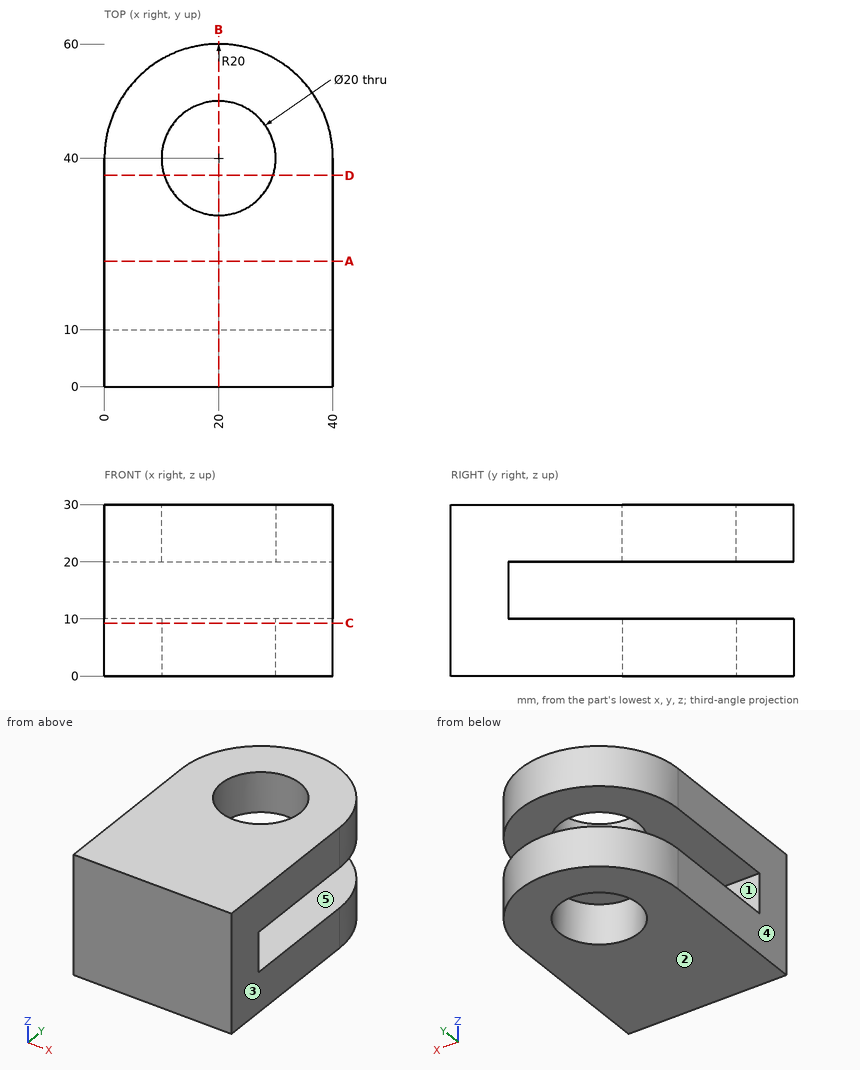
Answer from the drawing. Dimensions are ordinates in mm from the lowest x, y and z of the part. A direction names the side the tool comes from. Round coordinates to 2 decimals unless told otherwise and drop trailing zeros. Loops run counter-clockwise (first coordinate to the right, second up) from the corner with the lowest first, then second, coordinate; pieces in that order, holes last.
Q1. Section A-A on y = 22 is taken. Write down the section's boundary in (x, z).
Q2. Determine the mould class of the marked faces 1, 2 and 3 for opening direction Z: released by +Z, released by -Z, zero draft, split by the parting line, or undercut.
Q3. Consider probe 1 along Z at (x, y) = (21.5, 12); probe 2 along Y at (x, z) = (20, 4.75); probe 3 along X at (y, z) = (35.5, 21.25). Determine where each line is inside the solid, lowest interval first.
Q4. Section B-B on x = 20 is taken. Write down the section's boundary in (y, z).
Q5. Which of the six approach directions +Z, -Z, +X, -X, +Y, -Y give full straight-line access (tool end or side, diameter ignored) to the marked faces 4 and 5?
Q6. Section D-D on y = 37 is taken. Write down the section's boundary in (x, z), and give its area (3 significant figures).
Q7. Section C-C on z = 9.25 is taken. Write down the section's boundary in (x, y), and give its area (3 significant figures).
Q8. Each of these flat-tipped pins is pushed along its axis until it touches: pin 1 (12 mm diameter, centred on x = 20, y = 40, fed in from +Z); pin 2 (8 mm diameter, centred on x = 23.5, z = 15.5, fed in from +Y); pin 3 (10 mm diameter, centred on x = 16.5, z = 26, fed in from +Y). Where does it stop, or does it pass through?
Output:
1. outline: (0, 0) - (40, 0) - (40, 10) - (0, 10) - close; (0, 20) - (40, 20) - (40, 30) - (0, 30) - close
2. face 1: undercut
2. face 2: released by -Z
2. face 3: zero draft
3. probe 1: z = 0 to 10, 20 to 30
3. probe 2: y = 0 to 30, 50 to 60
3. probe 3: x = 0 to 11.07, 28.93 to 40
4. outline: (0, 0) - (30, 0) - (30, 10) - (10, 10) - (10, 20) - (30, 20) - (30, 30) - (0, 30) - close; (50, 0) - (60, 0) - (60, 10) - (50, 10) - close; (50, 20) - (60, 20) - (60, 30) - (50, 30) - close
5. face 4: +Z, -Z, -X, +Y, -Y
5. face 5: +X, -X, +Y
6. outline: (0, 0) - (10.46, 0) - (10.46, 10) - (0, 10) - close; (0, 20) - (10.46, 20) - (10.46, 30) - (0, 30) - close; (29.54, 0) - (40, 0) - (40, 10) - (29.54, 10) - close; (29.54, 20) - (40, 20) - (40, 30) - (29.54, 30) - close
6. area: 418 mm2
7. outline: (0, 0) - (40, 0) - (40, 40) arc R20 ccw to (0, 40) - close; hole circle Ø20 at (20, 40)
7. area: 1,910 mm2
8. pin 1: passes through
8. pin 2: stops at y = 10
8. pin 3: stops at y = 60
